from build123d import *

# Parameters (mm, degrees)
PAD001_DEPTH = 2.5
SKETCH_R     = 55
PAD_DEPTH    = 25
POCKET_DEPTH = 25
FILLET_R     = 8
CHAMFER_SIZE = 5


with BuildPart() as part:
    # Sketch001 → Pad001 (new body)
    with BuildSketch(Plane.XY):
        with BuildLine():
            ThreePointArc((38.890873, 38.890873), (27.935891, 67.443206), (0, 55))
            ThreePointArc((0, 55), (-27.935891, 67.443206), (-38.890873, 38.890873))
            ThreePointArc((-38.890873, 38.890873), (-67.443206, 27.935891), (-55, 0))
            ThreePointArc((-55, 0), (-67.443206, -27.935891), (-38.890873, -38.890873))
            ThreePointArc((-38.890873, -38.890873), (-27.935891, -67.443206), (0, -55))
            ThreePointArc((0, -55), (27.935891, -67.443206), (38.890873, -38.890873))
            ThreePointArc((38.890873, -38.890873), (67.443206, -27.935891), (55, 0))
            ThreePointArc((55, 0), (67.443206, 27.935891), (38.890873, 38.890873))
        make_face()
    extrude(amount=PAD001_DEPTH)

    # Sketch (on Face10 of Pad001) → Pad (join)
    with BuildSketch(Plane.XY.offset(2.5)):
        Circle(SKETCH_R)
    extrude(amount=PAD_DEPTH)

    # Sketch002 (on Face19 of Pad) → Pocket (cut)
    with BuildSketch(Plane.XY.offset(27.5)):
        with BuildLine():
            Line((10.937159, -51.348112), (11.457976, -53.79326))
            ThreePointArc((11.457976, -53.79326), (21.047589, -50.813374), (29.935566, -46.139591))
            Line((28.574859, -44.042337), (29.935566, -46.139591))
            ThreePointArc((28.574859, -44.042337), (48.503675, 20.09088), (-10.937159, 51.348112))
            Line((-11.457976, 53.79326), (-10.937159, 51.348112))
            ThreePointArc((-11.457976, 53.79326), (-21.047589, 50.813374), (-29.935566, 46.139591))
            Line((-29.935566, 46.139591), (-28.574859, 44.042337))
            ThreePointArc((-28.574859, 44.042337), (-48.503675, -20.09088), (10.937159, -51.348112))
        make_face()
    extrude(amount=-POCKET_DEPTH, mode=Mode.SUBTRACT)

    # Fillet
    fillet_edges = [part.edges().sort_by_distance(p)[0] for p in [
        (-29.255213, 45.090964, 27.5),
        (-11.197567, 52.570686, 27.5),
        (11.197567, -52.570686, 27.5),
        (29.255213, -45.090964, 27.5),
    ]]
    fillet(fillet_edges, radius=FILLET_R)

    # Chamfer
    chamfer_edges = [part.edges().sort_by_distance(p)[0] for p in [
        (-48.503675, -20.09088, 2.5),
        (48.503675, 20.09088, 2.5),
    ]]
    chamfer(chamfer_edges, length=CHAMFER_SIZE)


solid = part.part
Source: CAD feature listing. Evaluate the final solid. Frame: model axes, mm. A direction names the side the tool comes from. Round coordinates to 2 decimals unless told otherwise and drop trailing zeros. Order: outer loops, then holes, each group sorted by start corner. A loop starts at its lowest first (then second) coordinate and runs counter-clockwise, first axis right, second up. Notation, with made-up numbers: (-22, 10) - (28, 10) arc R27 cw to (28, 27) - close; hole circle Ø3 at (0, -9.75). An arc over 180 degrees is marked (long way). Use a Markdown table: item, result. Add a question column.
1. Section query A-A (z = 12.75). Return the cut outline in (x, y), then the cut area to 3 significant figures.
2. Line query: probe 1 along Z at (x, y) = (-34.5, -51.5); probe 2 along X at (y, z) = (-1.5, 18.25); probe 3 along X at (y, z) = (-45.5, 8.25). Output: solid intervals per line, ascending.
3. Section query B-B (z = 4.25). Return the cut outline in (x, y), then the cut area to 3 significant figures.
4. First-contact query: pin 1 (1 mm diameter, centred on y = 12.5, z = 8.5, fed in from +X); pin 2 (1 mm diameter, centred on y = 20, z = 12, fed in from +X); pin 3 (1.5 mm diameter, centred on x = -45, y = -3, fed in from +Z). Flat tips, straight axial feed; report the tip coordinate or a pass-through.
5. Set-up query: faces 1 (the flat face through (11.013, -51.704, 9.23)), 2 (the flat face through (-28.83, 44.436, 9.23)), 3 (the flat face through (-1, 1, 2.5)), 4 (the flat face through (28.773, -44.348, 9.23)), 5 (the flat face through (-25, -57, 2.5)). Return all of +Z, -Z, +X, -X, +Y, -Y with unobstructed straight access to the full face (end or side cutting, diameter ignored); none if empty.
Derived:
| question | item | result |
|---|---|---|
| 1 | outline | (-29.94, 46.14) arc R55 ccw to (11.46, -53.79) - (10.94, -51.35) arc R52.5 cw to (-28.57, 44.04) - close; (-11.46, 53.79) - (-10.94, 51.35) arc R52.5 cw to (28.57, -44.04) - (29.94, -46.14) arc R55 ccw to start |
| 1 | area | 746 mm2 |
| 2 | probe 1 | 0 to 2.5 |
| 2 | probe 2 | -54.98 to -52.48, 52.48 to 54.98 |
| 2 | probe 3 | -30.9 to -26.19, 29.52 to 30.9 |
| 3 | outline | (-29.94, 46.14) arc R55 ccw to (11.46, -53.79) - (10.26, -48.17) arc R49.25 cw to (-26.81, 41.32) - close; (-11.46, 53.79) - (-10.26, 48.17) arc R49.25 cw to (26.81, -41.32) - (29.94, -46.14) arc R55 ccw to start |
| 3 | area | 1,660 mm2 |
| 4 | pin 1 | x = 53.67 |
| 4 | pin 2 | x = 51.43 |
| 4 | pin 3 | z = 2.5 |
| 5 | face 1 | +Z, +X |
| 5 | face 2 | +Z, +Y |
| 5 | face 3 | +Z |
| 5 | face 4 | +Z, -Y |
| 5 | face 5 | +Z, -X, -Y |
